Here's the drawing with two shaded views (mm, measured from the low corner). I have some questions. A direction names the side the tool comes from. Give positions to 0.01 mm unless a question says otherwise; leave off trailing zeros. Write each loop counter-clockwise with the first axis right and the second up, starting at its lowest first coordinate (ties: lowest second). Pieces come first, ordered by that corner, then holes.
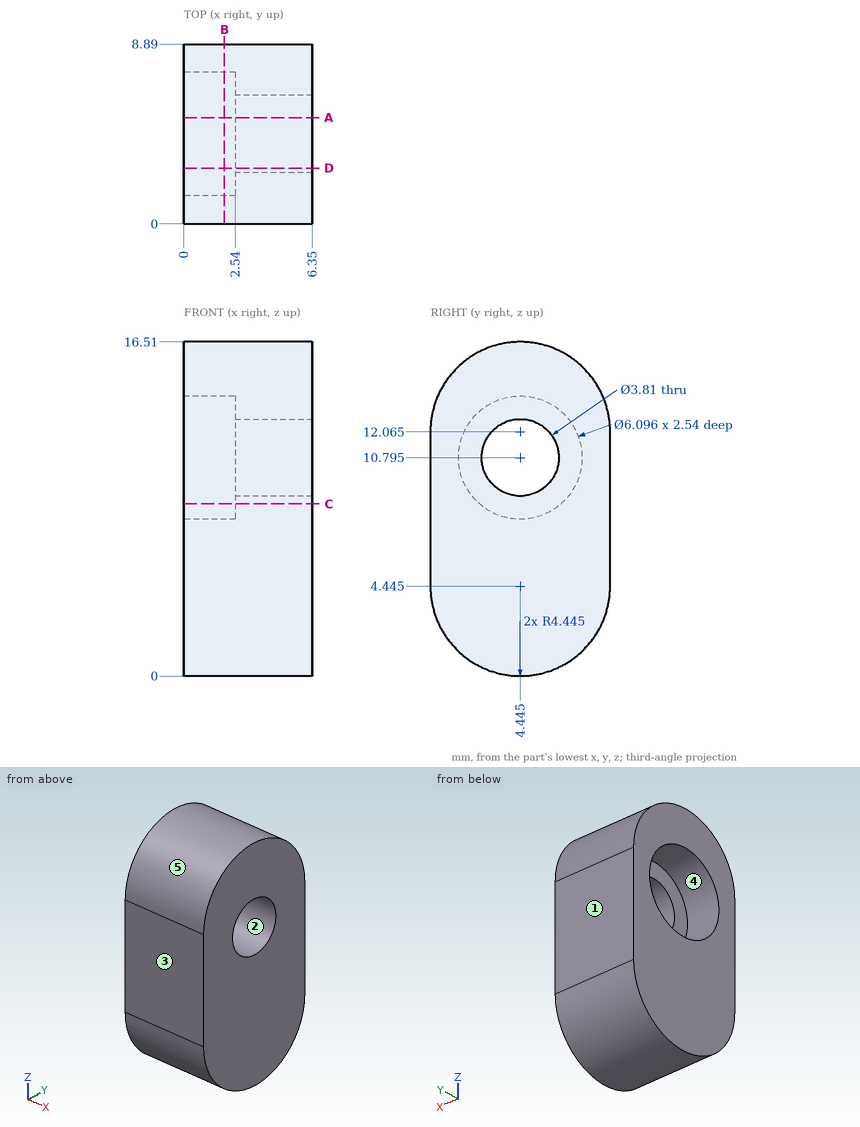
1) Suppose I cut it at B-B on x = 2. Write out the boundary of the cut face in (y, z) (3 decimals).
Values follow:
outline: (0, 4.445) arc R4.445 ccw to (8.89, 4.445) - (8.89, 12.065) arc R4.445 ccw to (0, 12.065) - close; hole circle Ø6.096 at (4.445, 10.795)
2) Please list where these lines run through material, in increasing order: L1, parallel to Z at x = 5, y = 4.25; L2, parallel to Z at x = 5.25, y = 3; L3, parallel to Y at x = 3.5, z = 10.5.
Values follow:
L1: z = 0 to 8.9, 12.69 to 16.51
L2: z = 0.24 to 9.55, 12.04 to 16.27
L3: y = 0 to 2.56, 6.33 to 8.89
3) For pin 1 Ø2 at (x, y) = (1, 7) entering from -Z; pin 2 Ø5 at (y, z) = (4.445, 10.795) entering from -X; pin 3 Ø1.5 at (x, y) = (4, 1) entering from -Z; pin 4 Ø2.5 at (y, z) = (4.445, 10.795) entering from -X, each with a flat end and sliding along its axis, tell me the tip position at first contact or that it passes through.
Values follow:
pin 1: stops at z = 0.28
pin 2: stops at x = 2.54
pin 3: stops at z = 0.91
pin 4: passes through
4) If we mould it in two halves opening along Y, with no side actions, what happens to the marked faces 1, 2 and 3? For each: +Y half, -Y half, draft (parallel to the pull), parting line (faces both ways), or undercut.
Values follow:
face 1: +Y half
face 2: undercut
face 3: -Y half
5) Suppose I cut it at D-D on y = 2.75. Write out the boundary of the cut face in (x, z).
Values follow:
outline: (0, 0.34) - (6.35, 0.34) - (6.35, 9.93) - (2.54, 9.93) - (2.54, 8.26) - (0, 8.26) - close; (0, 13.33) - (2.54, 13.33) - (2.54, 11.66) - (6.35, 11.66) - (6.35, 16.17) - (0, 16.17) - close
6) Suppose I cut it at A-A on y = 5.25. Write out the boundary of the cut face in (x, z).
Values follow:
outline: (0, 0.07) - (6.35, 0.07) - (6.35, 9.07) - (2.54, 9.07) - (2.54, 7.86) - (0, 7.86) - close; (0, 13.73) - (2.54, 13.73) - (2.54, 12.52) - (6.35, 12.52) - (6.35, 16.44) - (0, 16.44) - close
7) For the marked faces 4 and 5, which set-ups out of +Z, -Z, +X, -X, +Y, -Y let a thin tool reach every point of the face, with its end or its side?
Values follow:
face 4: -X
face 5: +Z, +X, -X
8) Suppose I cut it at C-C on z = 8.5. Write out the boundary of the cut face in (x, y).
Values follow:
outline: (0, 0) - (6.35, 0) - (6.35, 8.89) - (0, 8.89) - (0, 6.45) - (2.54, 6.45) - (2.54, 2.44) - (0, 2.44) - close
